```python
from build123d import *
from OCP.BRepFilletAPI import BRepFilletAPI_MakeChamfer

# Parameters (mm, degrees)
BOSS_EXTRUDE1_DEPTH = 12
SKETCH2_OUTSIDE_W   = 51.976
SKETCH2_OUTSIDE_H   = 55.304
SKETCH2_OUTSIDE_R   = 10.5
CUT_EXTRUDE1_DEPTH  = 10
CUT_EXTRUDE1_DRAFT  = -45
SKETCH3_OUTSIDE_W   = 51.976
SKETCH3_OUTSIDE_H   = 55.304
SKETCH3_OUTSIDE_R   = 10.5
CUT_EXTRUDE2_DEPTH  = 10
CUT_EXTRUDE2_DRAFT  = -45
CHAMFER2_SIZE       = 0.2
CHAMFER2_SIZE2      = 0.546410162
SKETCH5_R           = 3
CUT_EXTRUDE5_DEPTH  = 20


with BuildPart() as part:
    # Sketch1 → Boss-Extrude1 (new body)
    with BuildSketch(Plane.XY):
        Polygon((11.180698914, -6.634461418), (11.335961585, 6.365538582), (0.155262671, 13), (-11.180698914, 6.634461418), (-11.335961585, -6.365538582), (-0.155262671, -13), align=None)
    extrude(amount=BOSS_EXTRUDE1_DEPTH)


with BuildPart() as cut_extrude1_tool:
    # Sketch2 outside → Cut-Extrude1 (with draft: the straight prism first)
    with BuildSketch(Plane.XY.offset(12)):
        Rectangle(SKETCH2_OUTSIDE_W, SKETCH2_OUTSIDE_H)
        Circle(SKETCH2_OUTSIDE_R, mode=Mode.SUBTRACT)
    extrude(amount=-CUT_EXTRUDE1_DEPTH)
    # Cut-Extrude1: the draft: its side faces are tilted about the plane it starts from
    cut_extrude1_sides = [cut_extrude1_tool.faces().sort_by_distance(p)[0] for p in [
        (0, -27.652, 7),
        (25.988, 0, 7),
        (0, 27.652, 7),
        (-25.988, 0, 7),
        (-10.5, 0, 7),
    ]]
    draft(cut_extrude1_sides, Plane.XY.offset(12), CUT_EXTRUDE1_DRAFT)


with BuildPart() as part_1:
    add(part.part)

    # Cut-Extrude1: cut by cut_extrude1_tool
    add(cut_extrude1_tool.part, mode=Mode.SUBTRACT)


with BuildPart() as cut_extrude2_tool:
    # Sketch3 outside → Cut-Extrude2 (with draft: the straight prism first)
    with BuildSketch(Plane(origin=(0, 0, 0), x_dir=(-1, 0, 0), z_dir=(0, 0, -1))):
        Rectangle(SKETCH3_OUTSIDE_W, SKETCH3_OUTSIDE_H)
        Circle(SKETCH3_OUTSIDE_R, mode=Mode.SUBTRACT)
    extrude(amount=-CUT_EXTRUDE2_DEPTH)
    # Cut-Extrude2: the draft: its side faces are tilted about the plane it starts from
    cut_extrude2_sides = [cut_extrude2_tool.faces().sort_by_distance(p)[0] for p in [
        (0, -27.652, 5),
        (-25.988, 0, 5),
        (0, 27.652, 5),
        (25.988, 0, 5),
        (10.5, 0, 5),
    ]]
    draft(cut_extrude2_sides, Plane(origin=(0, 0, 0), x_dir=(-1, 0, 0), z_dir=(0, 0, -1)), CUT_EXTRUDE2_DRAFT)


with BuildPart() as part_2:
    add(part_1.part)

    # Cut-Extrude2: cut by cut_extrude2_tool
    add(cut_extrude2_tool.part, mode=Mode.SUBTRACT)

    # Chamfer2: one chamfer whose edges measure the first distance from different faces: ONE call of the kernel's chamfer builder (chamfer() names one face for all edges)
    chamfer2_edges_1 = [part_2.edges().sort_by_distance(p)[0] for p in [
        (11.335961585, 6.365538582, 6),
    ]]
    chamfer2_side_1 = [part_2.faces().sort_by_distance(p)[0] for p in [
        (11.258330249, -0.134461418, 6),
    ]]
    chamfer2_edges_2 = [part_2.edges().sort_by_distance(p)[0] for p in [
        (0.155262671, 13, 6),
    ]]
    chamfer2_side_2 = [part_2.faces().sort_by_distance(p)[0] for p in [
        (5.745612128, 9.682769291, 6),
    ]]
    chamfer2_edges_3 = [part_2.edges().sort_by_distance(p)[0] for p in [
        (-11.180698914, 6.634461418, 6),
    ]]
    chamfer2_side_3 = [part_2.faces().sort_by_distance(p)[0] for p in [
        (-5.512718121, 9.817230709, 6),
    ]]
    chamfer2_edges_4 = [part_2.edges().sort_by_distance(p)[0] for p in [
        (-11.335961585, -6.365538582, 6),
    ]]
    chamfer2_side_4 = [part_2.faces().sort_by_distance(p)[0] for p in [
        (-11.258330249, 0.134461418, 6),
    ]]
    chamfer2_edges_5 = [part_2.edges().sort_by_distance(p)[0] for p in [
        (-0.155262671, -13, 6),
    ]]
    chamfer2_side_5 = [part_2.faces().sort_by_distance(p)[0] for p in [
        (-5.745612128, -9.682769291, 6),
    ]]
    chamfer2_edges_6 = [part_2.edges().sort_by_distance(p)[0] for p in [
        (11.180698914, -6.634461418, 6),
    ]]
    chamfer2_side_6 = [part_2.faces().sort_by_distance(p)[0] for p in [
        (5.512718121, -9.817230709, 6),
    ]]
    chamfer2 = BRepFilletAPI_MakeChamfer(part_2.part.solid().wrapped)
    for e in chamfer2_edges_1:
        chamfer2.Add(CHAMFER2_SIZE, CHAMFER2_SIZE2, e.wrapped, chamfer2_side_1[0].wrapped)  # the first distance lies on this face
    for e in chamfer2_edges_2:
        chamfer2.Add(CHAMFER2_SIZE, CHAMFER2_SIZE2, e.wrapped, chamfer2_side_2[0].wrapped)  # the first distance lies on this face
    for e in chamfer2_edges_3:
        chamfer2.Add(CHAMFER2_SIZE, CHAMFER2_SIZE2, e.wrapped, chamfer2_side_3[0].wrapped)  # the first distance lies on this face
    for e in chamfer2_edges_4:
        chamfer2.Add(CHAMFER2_SIZE, CHAMFER2_SIZE2, e.wrapped, chamfer2_side_4[0].wrapped)  # the first distance lies on this face
    for e in chamfer2_edges_5:
        chamfer2.Add(CHAMFER2_SIZE, CHAMFER2_SIZE2, e.wrapped, chamfer2_side_5[0].wrapped)  # the first distance lies on this face
    for e in chamfer2_edges_6:
        chamfer2.Add(CHAMFER2_SIZE, CHAMFER2_SIZE2, e.wrapped, chamfer2_side_6[0].wrapped)  # the first distance lies on this face
    add(Compound.cast(chamfer2.Shape()), mode=Mode.REPLACE)

    # Sketch5 → Cut-Extrude5 (cut)
    with BuildSketch(Plane(origin=(0, 0, 0), x_dir=(-1, 0, 0), z_dir=(0, 0, -1))):
        Circle(SKETCH5_R)
    extrude(amount=-CUT_EXTRUDE5_DEPTH, mode=Mode.SUBTRACT)


solid = part_2.part
```
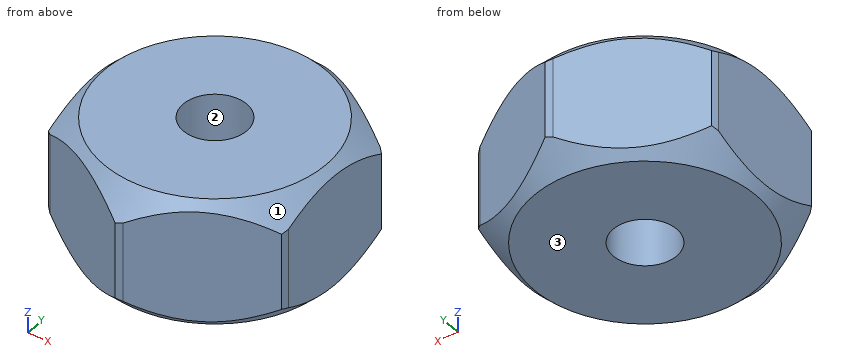
Model file for the job. Use its own axes, mm. Face numbers are marked on the shaded views. Round coordinates to 2 decimals unless told otherwise and drop trailing zeros. Order: outer loops, then holes, each group sorted by start corner. A loop starts at its lowest first (then second) coordinate and runs counter-clockwise, first axis right, second up. Notation, with made-up numbers: (4, -14) -> (43, -14) arc R9 cw to (43, -9) -> close; hole circle Ø5 at (72.5, 88). An arc over 180 degrees is marked (long way). Use one line per item in the form item = value.
Item 1: Cut at D-D, the plane z = 1.75. Write the cut outline in (x, y).
Returned:
outline = (-11.32, -4.69) arc R12.25 ccw to (-9.9, -7.22) -> (-1.59, -12.15) arc R12.25 ccw to (1.3, -12.18) -> (9.72, -7.45) arc R12.25 ccw to (11.2, -4.96) -> (11.32, 4.69) arc R12.25 ccw to (9.9, 7.22) -> (1.59, 12.15) arc R12.25 ccw to (-1.3, 12.18) -> (-9.72, 7.45) arc R12.25 ccw to (-11.2, 4.96) -> close; hole circle Ø6 at (0, 0)
Item 2: Drill centre lines: line 1 (Y direction, x = 2.25, z = 6.75); line 2 (Y direction, x = 0, z = 8.5); line 3 (X direction, y = -11.5, z = 7). Where is each one in solid material? Low to high.
Returned:
line_1 = -11.65 to -1.98, 1.98 to 11.76
line_2 = -12.81 to -3, 3 to 12.81
line_3 = -2.68 to 2.52
Item 3: Flat gauge pins, fed straight in: pin 1 Ø1 at (y, z) = (9.5, 3) entering from -X; pin 2 Ø5 at (y, z) = (8, 2) entering from -X; pin 3 Ø6 at (x, z) = (5.5, 7.5) entering from -Y. Where does each tip first touch, or does it go through?
Returned:
pin_1 = -6.97
pin_2 = -11.19
pin_3 = -11.51
Item 4: Pull direction Y, two halves, no side cores. Call the marked faces 1, 2 and 3: released by +Y, released by -Y, zero draft, split by the parting line, or undercut.
Returned:
face_1 = split by the parting line
face_2 = undercut
face_3 = zero draft
Item 5: Cut at C-C, the plane y = 0. Write the cut outline in (x, z), and give its area (3 significant figures).
Returned:
outline = (-11.26, 0.76) -> (-10.5, 0) -> (-3, 0) -> (-3, 12) -> (-10.5, 12) -> (-11.26, 11.24) -> close; (3, 0) -> (10.5, 0) -> (11.26, 0.76) -> (11.26, 11.24) -> (10.5, 12) -> (3, 12) -> close
area = 197 mm^2
Item 6: Cut at B-B, the plane x = 0. Write the cut outline in (y, z).
Returned:
outline = (-12.81, 2.31) -> (-10.5, 0) -> (-3, 0) -> (-3, 12) -> (-10.5, 12) -> (-12.81, 9.69) -> close; (3, 0) -> (10.5, 0) -> (12.81, 2.31) -> (12.81, 9.69) -> (10.5, 12) -> (3, 12) -> close
Item 7: Cut at A-A, the plane z = 4.5. Write the cut outline in (x, y).
Returned:
outline = (-11.33, -6.17) -> (-10.87, -6.64) -> (-0.33, -12.9) -> (0.32, -12.73) -> (11.01, -6.73) -> (11.19, -6.09) -> (11.33, 6.17) -> (10.87, 6.64) -> (0.33, 12.9) -> (-0.32, 12.73) -> (-11.01, 6.73) -> (-11.19, 6.09) -> close; hole circle Ø6 at (0, 0)
